from build123d import *

# Parameters (mm, degrees)
SKETCH1_R           = 1.25
SKETCH1_W           = 22.9
SKETCH1_H           = 12.4
BOSS_EXTRUDE1_DEPTH = 15
SKETCH4_W           = 25
SKETCH4_H           = 36.5
BOSS_EXTRUDE2_DEPTH = 4
SKETCH3_R           = 1.25
CUT_EXTRUDE1_DEPTH  = 35.502452959
CHAMFER1_SIZE       = 0.5
FILLET1_R           = 1


with BuildPart() as part:
    # Sketch1 → Boss-Extrude1 (new body)
    with BuildSketch(Plane.XY):
        Polygon((16.45, -8.2), (16.45, 8.2), (-21.110341698, 8.2), (-21.110341698, 18.2), (-25.110341698, 18.2), (-25.110341698, -18.2), (-21.110341698, -18.2), (-21.110341698, -8.2), align=None)
        with Locations((13.18, 0)):
            Circle(SKETCH1_R, mode=Mode.SUBTRACT)
        with Locations((-13.18, 0)):
            Circle(SKETCH1_R, mode=Mode.SUBTRACT)
        Rectangle(SKETCH1_W, SKETCH1_H, mode=Mode.SUBTRACT)
    extrude(amount=BOSS_EXTRUDE1_DEPTH)

    # Sketch4 → Boss-Extrude2 (add)
    with BuildSketch(Plane.ZY.offset(25.110341698)):
        with Locations((2.5, -0.05)):
            Rectangle(SKETCH4_W, SKETCH4_H)
    extrude(amount=-BOSS_EXTRUDE2_DEPTH)

    # Sketch3 → Cut-Extrude1 (cut, through all)
    with BuildSketch(Plane(origin=(0, 0, 0), x_dir=(0, 0, -1), z_dir=(1, 0, 0))):
        with Locations((-8.75, 13.2)):
            Circle(SKETCH3_R)
        with Locations((3.75, 13.2)):
            Circle(SKETCH3_R)
        with Locations((3.75, -13.2)):
            Circle(SKETCH3_R)
        with Locations((-8.75, -13.2)):
            Circle(SKETCH3_R)
    extrude(amount=-CUT_EXTRUDE1_DEPTH, mode=Mode.SUBTRACT)

    # Chamfer1
    # the kernel refuses this chamfer: 0.5 mm, written as the material it takes off along each edge
    with BuildSketch(Plane(origin=(-25.110341698, 19.485841494, 15), x_dir=(0.9996219169112968, 0, 0.02749587661058555), z_dir=(0, -1, 0))) as chamfer1_piece_1:
        Polygon((CHAMFER1_SIZE * 0.999621916911, -CHAMFER1_SIZE * 0.0274958766106), (-CHAMFER1_SIZE * 0.0274958766106, -CHAMFER1_SIZE * 0.999621916911), (0, 0), align=None)
    extrude(amount=39.071682988, mode=Mode.SUBTRACT)
    with BuildSketch(Plane(origin=(11.45, -6.2, 15), x_dir=(0.9996219169112968, 0, 0.02749587661058574), z_dir=(0, 1, 0)), Plane(origin=(-11.45, 6.2, 15), x_dir=(-0.9996219169112968, 0, 0.027495876610585647), z_dir=(0, -1, 0))) as chamfer1_piece_2:
        Polygon((CHAMFER1_SIZE * 0.999621916911, CHAMFER1_SIZE * 0.0274958766106), (-CHAMFER1_SIZE * 0.0274958766106, CHAMFER1_SIZE * 0.999621916911), (0, 0), align=None)
    extrude(amount=12.4, mode=Mode.SUBTRACT)
    with BuildSketch(Plane(origin=(11.45, 6.2, 15), x_dir=(0, 0.9996219169112968, 0.027495876610585647), z_dir=(-1, 0, 0)), Plane(origin=(-11.45, -6.2, 15), x_dir=(0, -0.9996219169112968, 0.027495876610585647), z_dir=(1, 0, 0))) as chamfer1_piece_3:
        Polygon((CHAMFER1_SIZE * 0.999621916911, CHAMFER1_SIZE * 0.0274958766106), (-CHAMFER1_SIZE * 0.0274958766106, CHAMFER1_SIZE * 0.999621916911), (0, 0), align=None)
    extrude(amount=22.9, mode=Mode.SUBTRACT)
    with BuildSketch(Plane(origin=(13.18, 0, 15), x_dir=(1, 0, 0), z_dir=(0, -1, 0))) as chamfer1_piece_4:
        Polygon((1.25 + CHAMFER1_SIZE, 0), (1.25, -CHAMFER1_SIZE), (1.25, 0), align=None)
    revolve(axis=Axis((13.18, 0, 15), (0, 0, 1)), mode=Mode.SUBTRACT)
    with BuildSketch(Plane(origin=(-13.18, 0, 15), x_dir=(1, 0, 0), z_dir=(0, -1, 0))) as chamfer1_piece_5:
        Polygon((1.25 + CHAMFER1_SIZE, 0), (1.25, -CHAMFER1_SIZE), (1.25, 0), align=None)
    revolve(axis=Axis((-13.18, 0, 15), (0, 0, 1)), mode=Mode.SUBTRACT)
    with BuildSketch(Plane(origin=(11.45, -7.485841494, 15), x_dir=(0.9996219169112968, 0, 0.027495876610585647), z_dir=(0, 1, 0))) as chamfer1_piece_6a_section:
        Polygon((CHAMFER1_SIZE * 0.999621916911, CHAMFER1_SIZE * 0.0274958766106), (-CHAMFER1_SIZE * 0.0274958766106, CHAMFER1_SIZE * 0.999621916911), (0, 0), align=None)
    chamfer1_piece_6a = extrude(amount=13.685841494, mode=Mode.PRIVATE)
    chamfer1_piece_6a = split(chamfer1_piece_6a, bisect_by=Plane(origin=(11.614896813, -6.2, 14.835103187), z_dir=(0, -1, 0)), keep=Keep.TOP, mode=Mode.PRIVATE)
    with BuildSketch(Plane(origin=(-11.45, -6.2, 15), x_dir=(0, -0.9996219169112968, 0.027495876610585647), z_dir=(1, 0, 0))) as chamfer1_piece_6b_section:
        Polygon((CHAMFER1_SIZE * 0.999621916911, CHAMFER1_SIZE * 0.0274958766106), (-CHAMFER1_SIZE * 0.0274958766106, CHAMFER1_SIZE * 0.999621916911), (0, 0), align=None)
    chamfer1_piece_6b = extrude(amount=24.185841494, mode=Mode.PRIVATE)
    chamfer1_piece_6b = split(chamfer1_piece_6b, bisect_by=Plane(origin=(11.45, -6.364896813, 14.835103187), z_dir=(1, 0, 0)), keep=Keep.TOP, mode=Mode.PRIVATE)
    chamfer1_piece_6 = chamfer1_piece_6a & chamfer1_piece_6b
    add(chamfer1_piece_6, mode=Mode.SUBTRACT)
    with BuildSketch(Plane(origin=(11.45, -6.2, 15), x_dir=(0.9996219169112968, 0, 0.02749587661058574), z_dir=(0, 1, 0))) as chamfer1_piece_7a_section:
        Polygon((CHAMFER1_SIZE * 0.999621916911, CHAMFER1_SIZE * 0.0274958766106), (-CHAMFER1_SIZE * 0.0274958766106, CHAMFER1_SIZE * 0.999621916911), (0, 0), align=None)
    chamfer1_piece_7a = extrude(amount=13.685841494, mode=Mode.PRIVATE)
    chamfer1_piece_7a = split(chamfer1_piece_7a, bisect_by=Plane(origin=(11.614896813, 6.2, 14.835103187), z_dir=(0, 1, 0)), keep=Keep.TOP, mode=Mode.PRIVATE)
    with BuildSketch(Plane(origin=(12.735841494, 6.2, 15), x_dir=(0, 0.9996219169112968, 0.027495876610585647), z_dir=(-1, 0, 0))) as chamfer1_piece_7b_section:
        Polygon((CHAMFER1_SIZE * 0.999621916911, CHAMFER1_SIZE * 0.0274958766106), (-CHAMFER1_SIZE * 0.0274958766106, CHAMFER1_SIZE * 0.999621916911), (0, 0), align=None)
    chamfer1_piece_7b = extrude(amount=24.185841494, mode=Mode.PRIVATE)
    chamfer1_piece_7b = split(chamfer1_piece_7b, bisect_by=Plane(origin=(11.45, 6.364896813, 14.835103187), z_dir=(1, 0, 0)), keep=Keep.TOP, mode=Mode.PRIVATE)
    chamfer1_piece_7 = chamfer1_piece_7a & chamfer1_piece_7b
    add(chamfer1_piece_7, mode=Mode.SUBTRACT)
    with BuildSketch(Plane(origin=(-11.45, 7.485841494, 15), x_dir=(-0.9996219169112968, 0, 0.027495876610585647), z_dir=(0, -1, 0))) as chamfer1_piece_8a_section:
        Polygon((CHAMFER1_SIZE * 0.999621916911, CHAMFER1_SIZE * 0.0274958766106), (-CHAMFER1_SIZE * 0.0274958766106, CHAMFER1_SIZE * 0.999621916911), (0, 0), align=None)
    chamfer1_piece_8a = extrude(amount=13.685841494, mode=Mode.PRIVATE)
    chamfer1_piece_8a = split(chamfer1_piece_8a, bisect_by=Plane(origin=(-11.614896813, 6.2, 14.835103187), z_dir=(0, 1, 0)), keep=Keep.TOP, mode=Mode.PRIVATE)
    with BuildSketch(Plane(origin=(11.45, 6.2, 15), x_dir=(0, 0.9996219169112968, 0.027495876610585647), z_dir=(-1, 0, 0))) as chamfer1_piece_8b_section:
        Polygon((CHAMFER1_SIZE * 0.999621916911, CHAMFER1_SIZE * 0.0274958766106), (-CHAMFER1_SIZE * 0.0274958766106, CHAMFER1_SIZE * 0.999621916911), (0, 0), align=None)
    chamfer1_piece_8b = extrude(amount=24.185841494, mode=Mode.PRIVATE)
    chamfer1_piece_8b = split(chamfer1_piece_8b, bisect_by=Plane(origin=(-11.45, 6.364896813, 14.835103187), z_dir=(-1, 0, 0)), keep=Keep.TOP, mode=Mode.PRIVATE)
    chamfer1_piece_8 = chamfer1_piece_8a & chamfer1_piece_8b
    add(chamfer1_piece_8, mode=Mode.SUBTRACT)
    with BuildSketch(Plane(origin=(-12.735841494, -6.2, 15), x_dir=(0, -0.9996219169112968, 0.027495876610585647), z_dir=(1, 0, 0))) as chamfer1_piece_9a_section:
        Polygon((CHAMFER1_SIZE * 0.999621916911, CHAMFER1_SIZE * 0.0274958766106), (-CHAMFER1_SIZE * 0.0274958766106, CHAMFER1_SIZE * 0.999621916911), (0, 0), align=None)
    chamfer1_piece_9a = extrude(amount=24.185841494, mode=Mode.PRIVATE)
    chamfer1_piece_9a = split(chamfer1_piece_9a, bisect_by=Plane(origin=(-11.45, -6.364896813, 14.835103187), z_dir=(-1, 0, 0)), keep=Keep.TOP, mode=Mode.PRIVATE)
    with BuildSketch(Plane(origin=(-11.45, 6.2, 15), x_dir=(-0.9996219169112968, 0, 0.027495876610585647), z_dir=(0, -1, 0))) as chamfer1_piece_9b_section:
        Polygon((CHAMFER1_SIZE * 0.999621916911, CHAMFER1_SIZE * 0.0274958766106), (-CHAMFER1_SIZE * 0.0274958766106, CHAMFER1_SIZE * 0.999621916911), (0, 0), align=None)
    chamfer1_piece_9b = extrude(amount=13.685841494, mode=Mode.PRIVATE)
    chamfer1_piece_9b = split(chamfer1_piece_9b, bisect_by=Plane(origin=(-11.614896813, -6.2, 14.835103187), z_dir=(0, -1, 0)), keep=Keep.TOP, mode=Mode.PRIVATE)
    chamfer1_piece_9 = chamfer1_piece_9a & chamfer1_piece_9b
    add(chamfer1_piece_9, mode=Mode.SUBTRACT)

    # Fillet1
    fillet1_edges = [part.edges().sort_by_distance(p)[0] for p in [
        (-21.110341698, -13.25, 15),
        (-21.110341698, 0, 0),
        (-21.110341698, 13.2, 15),
        (-21.110341698, -8.2, 7.5),
        (-2.330170849, -8.2, 15),
        (-2.330170849, -8.2, 0),
        (-2.330170849, 8.2, 15),
        (-21.110341698, 8.2, 7.5),
        (-2.330170849, 8.2, 0),
        (16.45, -8.2, 7.5),
        (16.45, 0, 15),
        (16.45, 8.2, 7.5),
        (16.45, 0, 0),
        (-21.110341698, 18.2, 2.5),
        (-22.860341698, 18.2, 15),
        (-23.110341698, -18.3, -10),
        (-23.110341698, 18.2, -10),
        (-21.110341698, -0.05, -10),
        (-22.860341698, -18.3, 15),
        (-21.110341698, -18.3, 2.5),
    ]]
    fillet(fillet1_edges, radius=FILLET1_R)


solid = part.part
Source: CAD feature listing. Evaluate the final solid. Frame: model axes, mm. A direction names the side the tool comes from. Coordinates: 2 decimals unless noted, no trailing zeros. Loops run counter-clockwise (first coordinate to the right, second up) from the corner with the lowest first, then second, coordinate; pieces in that order, holes last. Notation, with made-up numbers: (25.25, 23.5) - (43.25, 23.5) arc R28 ccw to (43.25, 61.5) - close; hole circle Ø9 at (5, 54). An arc over 180 degrees is marked (long way). Return JSON: item names as keys, results as strings.
Q1. Section C-C, the plane z = -3.75. Return loops of the section in (x, y), plus the area to 3 significant figures.
Results:
{"outline": "(-25.11, -18.3) - (-22.11, -18.3) arc R1 ccw to (-21.11, -17.3) - (-21.11, -14.45) - (-25.11, -14.45) - close; (-25.11, -11.95) - (-21.11, -11.95) - (-21.11, 11.95) - (-25.11, 11.95) - close; (-25.11, 14.45) - (-21.11, 14.45) - (-21.11, 17.2) arc R1 ccw to (-22.11, 18.2) - (-25.11, 18.2) - close", "area": "126 mm2"}
Q2. Access query for faces 4 (the flat face through (-2, 8.2, 7)), 5 (the cylindrical face through (-2.579, 7.899, 0.285)), 6 (the cylindrical face through (-21.396, 13.256, 14.699)). Directions: +Z, -Z, +X, -X, +Y, -Y. A direction counts if a zero-diameter tool reaches every point of the face in a straight line with its end or side. Return the directions, or none.
Results:
{"face 4": "+Z, -Z, +X, +Y", "face 5": "-Z, +X, +Y", "face 6": "+Z, +X, +Y"}
Q3. Section A-A, the plane z = 8. Return loops of the section in (x, y), plus the area to 3 significant figures.
Results:
{"outline": "(-25.11, -18.3) - (-22.11, -18.3) arc R1 ccw to (-21.11, -17.3) - (-21.11, -14.2) - (-25.11, -14.2) - close; (-25.11, -12.2) - (-21.11, -12.2) - (-21.11, -9.2) arc R1 cw to (-20.11, -8.2) - (15.45, -8.2) arc R1 ccw to (16.45, -7.2) - (16.45, 7.2) arc R1 ccw to (15.45, 8.2) - (-20.11, 8.2) arc R1 cw to (-21.11, 9.2) - (-21.11, 12.2) - (-25.11, 12.2) - close; (-25.11, 14.2) - (-21.11, 14.2) - (-21.11, 17.2) arc R1 ccw to (-22.11, 18.2) - (-25.11, 18.2) - close; hole circle Ø2.5 at (-13.18, 0); hole (-11.45, -6.2) - (11.45, -6.2) - (11.45, 6.2) - (-11.45, 6.2) - close; hole circle Ø2.5 at (13.18, 0)", "area": "452 mm2"}
Q4. Section D-D, the plane y = 0. Return loops of the section in (x, z).
Results:
{"outline": "(-25.11, -10) - (-22.11, -10) arc R1 ccw to (-21.11, -9) - (-21.11, -1) arc R1 cw to (-20.11, 0) - (-14.43, 0) - (-14.43, 14.5) - (-14.93, 15) - (-24.61, 15) - (-25.11, 14.5) - close; (-11.93, 0) - (-11.45, 0) - (-11.45, 14.5) - (-11.69, 14.74) - (-11.93, 14.5) - close; (11.45, 0) - (11.93, 0) - (11.93, 14.5) - (11.69, 14.74) - (11.45, 14.5) - close; (14.43, 0) - (15.45, 0) arc R1 ccw to (16.45, 1) - (16.45, 14) arc R1 ccw to (15.45, 15) - (14.93, 15) - (14.43, 14.5) - close"}
Q5. Contact query for flat-ended pins moving along their axis: P1, Ø4.5, axis at x = 4, y = 2, coming from the -Z side; P2, Ø6, axis at x = -0.5, z = -2, coming from the -Y side; P3, Ø4.5, axis at x = 5, z = 7.5, coming from the +Y side; P4, Ø10, axis at x = -7, y = 2, coming from the -Z side. Output: stop coordinate, or through.
Results:
{"P1": "through", "P2": "y = -8.2", "P3": "y = 8.2", "P4": "z = 0"}
Q6. Section B-B, the plane y = -4. Return loops of the section in (x, z), plus the area to 3 significant figures.
Results:
{"outline": "(-25.11, -10) - (-22.11, -10) arc R1 ccw to (-21.11, -9) - (-21.11, -1) arc R1 cw to (-20.11, 0) - (-11.45, 0) - (-11.45, 14.5) - (-11.95, 15) - (-24.61, 15) - (-25.11, 14.5) - close; (11.45, 0) - (15.45, 0) arc R1 ccw to (16.45, 1) - (16.45, 14) arc R1 ccw to (15.45, 15) - (11.95, 15) - (11.45, 14.5) - close", "area": "319 mm2"}
Q7. Mould query, pull axis X, two halves, no side actions, for faces 1 (the cylindrical face through (-23.08, -13.15, 10)), 2 (the cylindrical face through (16.165, 7.899, 7.591)), 3 (the cylindrical face through (14.335, -0.479, 7.148)). Classes: released by +X, released by -X, zero draft, split by the parting line, or undercut.
Results:
{"face 1": "zero draft", "face 2": "released by +X", "face 3": "undercut"}
Q8. Material intervals for line 1 along Y through (x, z) = (-23.7, 8.75); line 2 along Y through (x, z) = (11, 4); line 3 along Y through (x, z) = (13.18, 4.25), sorted ascending.
Results:
{"line 1": "-18.3 to -14.45, -11.95 to 11.95, 14.45 to 18.2", "line 2": "-8.2 to -6.2, 6.2 to 8.2", "line 3": "-8.2 to -1.25, 1.25 to 8.2"}
